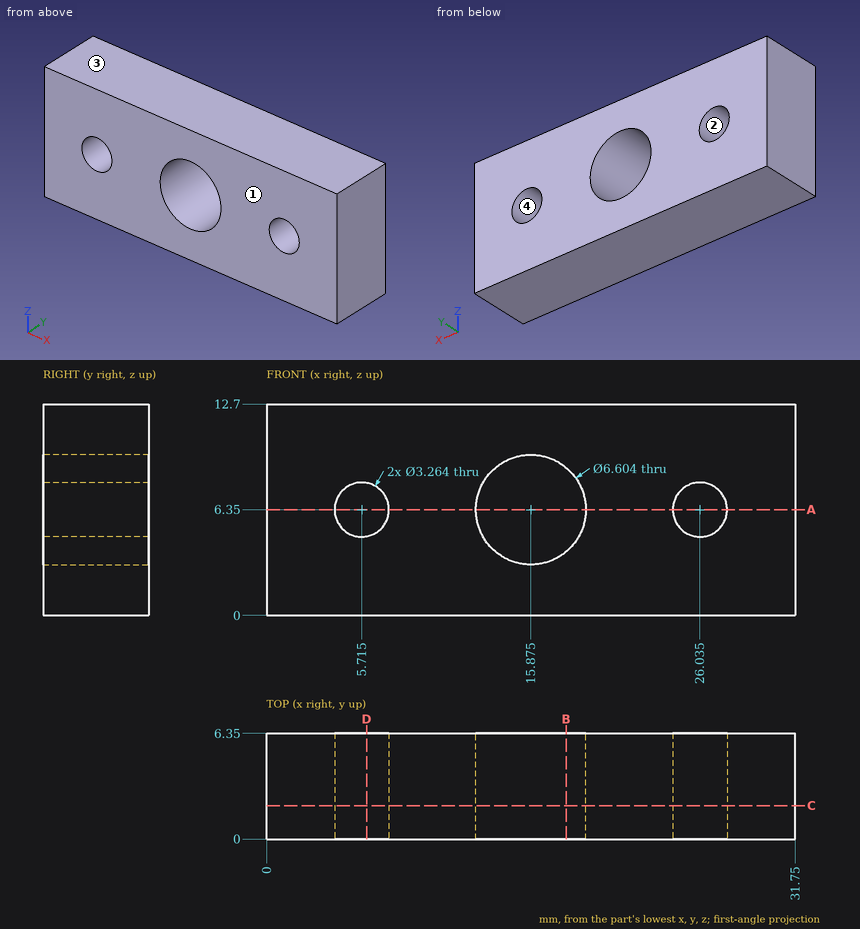
Input: dimensioned drawing with shaded views. Units: mm. Origin: part minimum x, y, z. Coordinates: 2 decimals unless noted, no trailing zeros. Order: outer loops, then holes, each group sorted by start corner. A loop starts at its lowest first (then second) coordinate and runs counter-clockwise, first axis right, second up. Notation, with made-up numbers: (73.25, 65.25) -> (82.25, 65.25) arc R29 ccw to (82.25, 98.25) -> close; hole circle Ø5 at (44.5, -22). An arc over 180 degrees is marked (long way). Use CSV: the item, a comma, the result in double quotes.
1) Section C-C on y = 2. Output: boundary loops of the cut face in (x, z) (3 decimals).
Findings:
outline,"(0, 0) -> (31.75, 0) -> (31.75, 12.7) -> (0, 12.7) -> close; hole circle Ø3.264 at (5.715, 6.35); hole circle Ø6.604 at (15.875, 6.35); hole circle Ø3.264 at (26.035, 6.35)"
2) Section D-D on x = 6. Output: boundary loops of the cut face in (y, z), then the cut area to 3 significant figures.
Findings:
outline,"(0, 0) -> (6.35, 0) -> (6.35, 4.74) -> (0, 4.74) -> close; (0, 7.96) -> (6.35, 7.96) -> (6.35, 12.7) -> (0, 12.7) -> close"
area,"60.2 mm^2"
3) Section A-A on z = 6.35. Output: boundary loops of the cut face in (x, y).
Findings:
outline,"(0, 0) -> (4.08, 0) -> (4.08, 6.35) -> (0, 6.35) -> close; (7.35, 0) -> (12.57, 0) -> (12.57, 6.35) -> (7.35, 6.35) -> close; (19.18, 0) -> (24.4, 0) -> (24.4, 6.35) -> (19.18, 6.35) -> close; (27.67, 0) -> (31.75, 0) -> (31.75, 6.35) -> (27.67, 6.35) -> close"
4) Line query: line 1 (Z direction, x = 26, y = 0.5); line 2 (X direction, y = 4, z = 6); line 3 (X direction, y = 1.75, z = 5). Output: solid intervals per line, ascending.
Findings:
line 1,"z = 0 to 4.72, 7.98 to 12.7"
line 2,"x = 0 to 4.12, 7.31 to 12.59, 19.16 to 24.44, 27.63 to 31.75"
line 3,"x = 0 to 4.8, 6.63 to 12.86, 18.89 to 25.12, 26.95 to 31.75"
5) Mould query, pull axis Z, two halves, no side actions, for the marked faces 1, 2, 3 and 4. Classes: +Z half, -Z half, draft (parallel to the pull), parting line (faces both ways), or undercut.
Findings:
face 1,"draft"
face 2,"undercut"
face 3,"+Z half"
face 4,"undercut"
6) Section B-B on x = 18. Output: boundary loops of the cut face in (y, z).
Findings:
outline,"(0, 0) -> (6.35, 0) -> (6.35, 3.82) -> (0, 3.82) -> close; (0, 8.88) -> (6.35, 8.88) -> (6.35, 12.7) -> (0, 12.7) -> close"
